from build123d import *

# Parameters (mm, degrees)
SKETCH4_R            = 55.88
BOSS_EXTRUDE2_DEPTH  = 10.16
BOSS_EXTRUDE4_DEPTH  = 101.6
BOSS_EXTRUDE5_DEPTH  = 9.525
BOSS_EXTRUDE6_START  = -9.525
BOSS_EXTRUDE6_DEPTH  = 9.525
CUT_EXTRUDE4_REACH   = 214.095
SKETCH12_R           = 20.828
SKETCH13_W           = 38.1
SKETCH13_H           = 69.85
CUT_EXTRUDE5_DEPTH   = 76.2
BOSS_EXTRUDE10_DEPTH = 19.05
SKETCH28_R           = 11.049
CUT_EXTRUDE9_DEPTH   = 38.1
CUT_EXTRUDE10_DEPTH  = 7.366
CHAMFER1_SIZE        = 6.35
SKETCH30_R           = 2.1
CUT_EXTRUDE11_DEPTH  = 7.366
SKETCH31_R           = 3.175
CUT_EXTRUDE12_DEPTH  = 215.41878972
BOSS_EXTRUDE11_DEPTH = 38.1
CHAMFER2_SIZE        = 25.4
CUT_EXTRUDE13_REACH  = 224.549
SKETCH34_R           = 3.175


with BuildPart() as part:
    # Sketch4 → Boss-Extrude2 (new body)
    with BuildSketch(Plane(origin=(0, 0, 0), x_dir=(1, 0, 0), z_dir=(0, 1, 0))):
        with Locations(Location((0, 0, 0), (0, 0, 270))):
            Circle(SKETCH4_R)
    extrude(amount=BOSS_EXTRUDE2_DEPTH)

    # Sketch8 → Boss-Extrude4 (add)
    with BuildSketch(Plane(origin=(0, 10.16, 0), x_dir=(1, 0, 0), z_dir=(0, 1, 0))):
        Polygon((0, 43.994090512), (-38.1, 21.997045256), (-38.1, -21.997045256), (0, -43.994090512), (38.1, -21.997045256), (38.1, 21.997045256), align=None)
    extrude(amount=BOSS_EXTRUDE4_DEPTH)

    # Sketch9 → Boss-Extrude5 (add)
    with BuildSketch(Plane(origin=(-19.05, 0, -32.995567884), x_dir=(-0.8660254037844386, 0, 0.5000000000000003), z_dir=(-0.5000000000000002, 0, -0.8660254037844385))):
        with BuildLine():
            Line((21.997045256, 111.76), (-21.997045256, 111.76))
            Line((-21.997045256, 111.76), (-21.997045256, 140.520185187))
            ThreePointArc((-21.997045256, 140.520185187), (0, 177.4), (21.997045256, 140.520185187))
            Line((21.997045256, 140.520185187), (21.997045256, 111.76))
        make_face()
    extrude(amount=-BOSS_EXTRUDE5_DEPTH)

    # Sketch10 → Boss-Extrude6 (add)
    with BuildSketch(Plane(origin=(19.05, 0, 32.995567884), x_dir=(0.8660254037844386, 0, -0.5000000000000001), z_dir=(0.5000000000000001, 0, 0.8660254037844386)).offset(BOSS_EXTRUDE6_START)):
        with BuildLine():
            Line((-21.997045256, 111.76), (21.997045256, 111.76))
            Line((21.997045256, 111.76), (21.997045256, 140.520185187))
            ThreePointArc((21.997045256, 140.520185187), (0, 177.4), (-21.997045256, 140.520185187))
            Line((-21.997045256, 140.520185187), (-21.997045256, 111.76))
        make_face()
    extrude(amount=BOSS_EXTRUDE6_DEPTH)

    # Cut-Extrude4: up to this face of the body (flat: up to its plane)
    cut_extrude4_end = Plane(part.part.faces().sort_by_distance((19.05, 92.730612225, 32.995567884))[0])
    # Sketch12 → Cut-Extrude4 (cut, up to the picked face)
    with BuildSketch(Plane(origin=(-19.05, 0, -32.995567884), x_dir=(-0.8660254037844386, 0, 0.5000000000000003), z_dir=(-0.5000000000000002, 0, -0.8660254037844385)), mode=Mode.PRIVATE) as cut_extrude4_sk1:
        with Locations((0, 152.4)):
            Circle(SKETCH12_R)
    cut_extrude4_tool1 = split(extrude(cut_extrude4_sk1.sketch, amount=-CUT_EXTRUDE4_REACH, mode=Mode.PRIVATE), bisect_by=cut_extrude4_end, keep=Keep.BOTH, mode=Mode.PRIVATE)
    add(cut_extrude4_tool1.solids().sort_by(Axis((-19.05, 152.4, -32.995568), (0.5000000000000002, 0, 0.8660254037844385)))[0], mode=Mode.SUBTRACT)

    # Sketch13 → Cut-Extrude5 (cut, symmetric)
    with BuildSketch(Plane(origin=(-19.05, 0, 10.998522628), x_dir=(0.5000000000000002, 0, 0.8660254037844386), z_dir=(-0.8660254037844385, 0, 0.5000000000000001))):
        with Locations((0, 76.835)):
            Rectangle(SKETCH13_W, SKETCH13_H)
    extrude(amount=CUT_EXTRUDE5_DEPTH, both=True, mode=Mode.SUBTRACT)

    # Sketch22 → Boss-Extrude10 (add, symmetric)
    with BuildSketch(Plane(origin=(0, 0, 0), x_dir=(-0.8660254037844386, 0, 0.5000000000000001), z_dir=(-0.5000000000000001, 0, -0.8660254037844386))):
        with BuildLine():
            Line((43.994090512, 41.91), (102.10102108, 41.91))
            ThreePointArc((102.10102108, 41.91), (117.97602108, 26.035), (102.10102108, 10.16))
            Line((102.10102108, 10.16), (43.994090512, 10.16))
            Line((43.994090512, 10.16), (21.997045256, 10.16))
            Line((21.997045256, 10.16), (21.997045256, 41.91))
            Line((21.997045256, 41.91), (43.994090512, 41.91))
        make_face()
    extrude(amount=BOSS_EXTRUDE10_DEPTH, both=True)

    # Sketch28 → Cut-Extrude9 (cut)
    with BuildSketch(Plane(origin=(9.525, 0, 16.497783942), x_dir=(0.8660254037844386, 0, -0.5000000000000001), z_dir=(0.5000000000000001, 0, 0.8660254037844386))):
        with Locations((-102.10102108, 26.035)):
            Circle(SKETCH28_R)
    extrude(amount=-CUT_EXTRUDE9_DEPTH, mode=Mode.SUBTRACT)

    # Sketch29 → Cut-Extrude10 (cut)
    with BuildSketch(Plane(origin=(9.525, 0, 16.497783942), x_dir=(0.8660254037844386, 0, -0.5000000000000001), z_dir=(0.5000000000000001, 0, 0.8660254037844386))):
        with BuildLine():
            Line((-115.737415068, 17.907), (-109.585405958, 17.907))
            ThreePointArc((-109.585405958, 17.907), (-113.15002108, 26.035), (-109.585405958, 34.163))
            Line((-109.585405958, 34.163), (-115.737415068, 34.163))
            ThreePointArc((-115.737415068, 34.163), (-117.97602108, 26.035), (-115.737415068, 17.907))
        make_face()
    extrude(amount=-CUT_EXTRUDE10_DEPTH, mode=Mode.SUBTRACT)

    # Chamfer1
    chamfer1_edges = [part.edges().sort_by_distance(p)[0] for p in [
        (38.1, 41.91, -10.998522628),
        (28.575, 41.91, -27.49630657),
    ]]
    chamfer(chamfer1_edges, length=CHAMFER1_SIZE)

    # Sketch30 → Cut-Extrude11 (cut)
    with BuildSketch(Plane(origin=(0, 41.91, 0), x_dir=(1, 0, 0), z_dir=(0, 1, 0))):
        with Locations(Location((-88.422078008, -51.05051054, 0), (0, 0, 270))):
            Circle(SKETCH30_R)
    extrude(amount=-CUT_EXTRUDE11_DEPTH, mode=Mode.SUBTRACT)

    # Sketch31 → Cut-Extrude12 (cut, through all)
    with BuildSketch(Plane(origin=(0, 10.16, 0), x_dir=(1, 0, 0), z_dir=(0, 1, 0))):
        with Locations(Location((-49.089000823, 6.594762938, 0), (0, 0, 270))):
            Circle(SKETCH31_R)
        with Locations(Location((26.925278647, 41.57222955, 0), (0, 0, 270))):
            Circle(SKETCH31_R)
    cut_extrude12 = extrude(amount=-CUT_EXTRUDE12_DEPTH, mode=Mode.SUBTRACT)

    # Mirror1: Cut-Extrude12 across plane
    add(cut_extrude12.mirror(Plane(origin=(0, 0, 0), x_dir=(-0.8660254037844386, 0, 0.5000000000000001), z_dir=(-0.5000000000000001, 0, -0.8660254037844386))), mode=Mode.SUBTRACT)

    # Sketch33 → Boss-Extrude11 (add)
    with BuildSketch(Plane(origin=(0, 41.91, 0), x_dir=(1, 0, 0), z_dir=(0, 1, 0))):
        with BuildLine():
            Line((-43.411916389, -22.079834386), (-63.092428819, -33.442383535))
            Line((-63.092428819, -33.442383535), (-61.800298466, -35.680418955))
            Line((-61.800298466, -35.680418955), (-60.542722832, -37.858603849))
            Line((-60.542722832, -37.858603849), (-40.91541904, -26.504074545))
            ThreePointArc((-40.91541904, -26.504074545), (-33.742060338, -19.539834386), (-43.411916389, -22.079834386))
        make_face()
    extrude(amount=BOSS_EXTRUDE11_DEPTH)

    # Chamfer2
    chamfer2_edges = [part.edges().sort_by_distance(p)[0] for p in [
        (-61.817575825, 80.01, 35.650493692),
    ]]
    chamfer(chamfer2_edges, length=CHAMFER2_SIZE)

    # Cut-Extrude13: up to this plane
    cut_extrude13_end = Plane(origin=(-60.542722832, 80.01, 37.858603849), z_dir=(-0.500750644235671, 0, -0.8655915851587056))
    # Sketch34 → Cut-Extrude13 (cut, up to the surface)
    with BuildSketch(Plane(origin=(-1.292130352, 0, -2.23803542), x_dir=(-0.8660254037844386, 0, 0.5000000000000003), z_dir=(-0.5000000000000002, 0, -0.8660254037844385)), mode=Mode.PRIVATE) as cut_extrude13_sk1:
        with Locations((55.184849848, 61.159110234)):
            Circle(SKETCH34_R)
    cut_extrude13_tool1 = split(extrude(cut_extrude13_sk1.sketch, amount=-CUT_EXTRUDE13_REACH, mode=Mode.PRIVATE), bisect_by=cut_extrude13_end, keep=Keep.BOTH, mode=Mode.PRIVATE)
    add(cut_extrude13_tool1.solids().sort_by_distance((-49.083612, 61.15911, 25.35439))[0], mode=Mode.SUBTRACT)


solid = part.part
Geometry: final body of the model. Coordinates: model frame, mm. A direction names the side the tool comes from. Give positions to 0.01 mm unless a question says otherwise; leave off trailing zeros. Loops run counter-clockwise (first coordinate to the right, second up) from the corner with the lowest first, then second, coordinate; pieces in that order, holes last. Notation, with made-up numbers: (-12.75, 87) -> (24.25, 87) arc R15 ccw to (24.25, 108) -> close; hole circle Ø6 at (8.25, -29). An arc over 180 degrees is marked (long way). Put each result on its own line as item: value.
1. Pin query (flat end, axial travel): P1, Ø6, axis at x = -11, y = 59, coming from the -Z side; P2, Ø13, axis at x = 6, z = 14.5, coming from the +Y side; P3, Ø10, axis at x = -43, y = 56.5, coming from the +Z side; P4, Ø1, axis at x = 5.5, z = 53, coming from the -Y side. Return the tip coordinate at first contact, or that it passes through.
Taken from the geometry:
P1: stops at z = -39.38
P2: stops at y = 111.76
P3: stops at z = 30.6
P4: stops at y = 0
2. Cut plane B-B (y = 68). Return the cut outline in (x, z).
Taken from the geometry:
outline: (-51.5, 26.75) -> (-43.41, 22.08) arc R5.17 ccw (long way) to (-40.92, 26.5) -> (-48.95, 31.15) -> close; (-38.1, -22) -> (0, -43.99) -> (19.05, -33) -> (-38.1, 0) -> close; (-19.05, 33) -> (38.1, 0) -> (38.1, 22) -> (0, 43.99) -> close
3. Set-up query: faces 4 (the flat face through (38.1, 49, 5)), 5 (the flat face through (-50.93, 55.44, 26.42)), 6 (the flat face through (-90, 34.163, 70)), 7 (the cylindrical face through (-33.65, 60.69, 19.71)). Return all of +Z, -Z, +X, -X, +Y, -Y with unobstructed straight access to the full face (end or side cutting, diameter ignored); none if empty.
Taken from the geometry:
face 4: +Z, -Z, +X
face 5: -Z, -X, +Y
face 6: +Z, +X
face 7: +Y
4. Cut plane A-A (y = 108). Return the cut outline in (x, z).
Taken from the geometry:
outline: (-38.1, -22) -> (0, -43.99) -> (19.05, -33) -> (-38.1, 0) -> close; (-19.05, 33) -> (38.1, 0) -> (38.1, 22) -> (0, 43.99) -> close
5. Cut plane C-C (y = 138). Return the cut outline in (x, z), plus the area to 3 significant figures.
Taken from the geometry:
outline: (-38.1, -22) -> (-32.08, -25.47) -> (-27.32, -17.22) -> (-33.34, -13.75) -> close; (-6.02, -40.52) -> (0, -43.99) -> (4.76, -35.75) -> (-1.26, -32.27) -> close; (-4.76, 35.75) -> (1.26, 32.27) -> (6.02, 40.52) -> (0, 43.99) -> close; (27.32, 17.22) -> (33.34, 13.75) -> (38.1, 22) -> (32.08, 25.47) -> close
area: 265 mm2
6. Pull-direction query (Z, two-part tool) for faces 1 (the cylindrical face through (52.565, 5.151, -3.22)), 2 (the flat face through (1, 0, -1)), 3 (the cylindrical face through (-102.3, 26.384, 58.755)); classes: released by +Z, released by -Z, zero draft, split by the parting line, or undercut.
Taken from the geometry:
face 1: undercut
face 2: zero draft
face 3: released by +Z
7. Ray query, line 1 along Y through (x, z) = (28, 6); line 2 along Y through (x, z) = (-21.5, -39); line 3 along Y through (x, z) = (-14, -31). Return the intervals inside material, ascending. Write a range as [from, to].
Taken from the geometry:
line 1: y = [0, 111.76]
line 2: y = [0, 10.16]
line 3: y = [0, 131.85], [172.95, 177.17]
